Input: part model. Units: mm. Frame: model coordinates. A direction names the side the tool comes from. Give positions to 0.01 mm unless a question says otherwise; leave off trailing zeros. Loops run counter-clockwise (first coordinate to the right, second up) from the corner with the lowest first, then second, coordinate; pieces in that order, holes last. Notation, with made-up numbers: M -3,54.25 L 48,54.25 A19 ccw 48,78.25 Z; hole C 9.5,22 d10. An arc over 180 degrees is marked long. Answer as a JSON object with one key per item and string values. Group by question number.
1) Section query D-D on x = -26. Return loops of the section in (y, z), plus the area to 3 significant figures.
2) First-contact query: P1, Ø6, axis at x = -50, z = 0, coming from the -Y side; P2, Ø4, axis at x = -20, z = 0, coming from the +Y side; P3, Ø3, axis at y = -20, z = 0, coming from the +X side. Flat tips, straight axial feed; report the tip coordinate or a pass-through.
3) Ray query, L1, parallel to Y at x = -10.5, z = 0; L2, parallel to Z at x = -20, y = -8.5; L3, parallel to Y at x = -9, z = -1.75. Return the intervals inside material, ascending.
4) Section query C-C on x = -32.5. Return loops of the section in (y, z), plus the area to 4 significant figures.
5) Section query B-B on z = 4. Return loops of the section in (x, y), plus the area to 3 significant figures.
6) Access query for faces 4 (the cylindrical face through (-7.6, -42.56, 0.54)), 5 (the flat face through (-40, -50, 0)), 6 (the cylindrical face through (-17.5, -7.6, -0.1)). Directions: +Z, -Z, +X, -X, +Y, -Y. A direction counts if a zero-diameter tool reaches every point of the face in a straight line with its end or side. Return the directions, or none.
7) Section query A-A on y = -7. Return loops of the section in (x, z), plus the area to 3 significant figures.
8) Draft query along Z for faces 1 (the flat face through (0, -30, 0)), 2 (the cylindrical face through (-7.6, -22.48, 0.33)), 3 (the flat face through (-30, -30, -5)). Return one class per face: +Z half, -Z half, draft (parallel to the pull), parting line (faces both ways), or undercut.
from build123d import *

# Parameters (mm, degrees)
EXTRUDE_1_DEPTH        = 5
HOLE_WIZARD_M6_1_D     = 5
HOLE_WIZARD_M6_1_DEPTH = 15
HOLE_WIZARD_M6_1_TIP   = 1.502151548
HOLE_WIZARD_M6_2_D     = 5
HOLE_WIZARD_M6_2_DEPTH = 15
HOLE_WIZARD_M6_2_TIP   = 1.502151548


with BuildPart() as part:
    # 草图1 → 凸台-拉伸1 (new body, symmetric)
    with BuildSketch(Plane.XY):
        Polygon((0, 0), (-60, 0), (-60, -40), (-20, -60), (0, -60), align=None)
    extrude(amount=EXTRUDE_1_DEPTH, both=True)

    # M6 螺纹孔1
    with Locations(Plane(origin=(0, -20, 0), x_dir=(0, 0, 1), z_dir=(1, 0, 0))):
        with Locations((0, 0), (0, 25)):
            Hole(HOLE_WIZARD_M6_1_D / 2, depth=HOLE_WIZARD_M6_1_DEPTH)
            with Locations((0, 0, -(HOLE_WIZARD_M6_1_DEPTH + HOLE_WIZARD_M6_1_TIP / 2))):  # 118° drill point
                Cone(0, HOLE_WIZARD_M6_1_D / 2, HOLE_WIZARD_M6_1_TIP, mode=Mode.SUBTRACT)

    # M6 螺纹孔2
    with Locations(Plane(origin=(-20, 0, 0), x_dir=(1, 0, 0), z_dir=(0, 1, 0))):
        with Locations((0, 0), (-30, 0)):
            Hole(HOLE_WIZARD_M6_2_D / 2, depth=HOLE_WIZARD_M6_2_DEPTH)
            with Locations((0, 0, -(HOLE_WIZARD_M6_2_DEPTH + HOLE_WIZARD_M6_2_TIP / 2))):  # 118° drill point
                Cone(0, HOLE_WIZARD_M6_2_D / 2, HOLE_WIZARD_M6_2_TIP, mode=Mode.SUBTRACT)


solid = part.part
Output:
{
 "1": {"outline": "M -57,-5 L 0,-5 L 0,5 L -57,5 Z", "area": "570 mm^2"},
 "2": {"P1": "stops at y = -46.5", "P2": "stops at y = -15.3", "P3": "stops at x = -15.6"},
 "3": {"L1": "y = -60 to -47.5, -42.5 to -22.5, -17.5 to 0", "L2": "z = -5 to -2.5, 2.5 to 5", "L3": "y = -60 to -46.79, -43.21 to -21.79, -18.21 to 0"},
 "4": {"outline": "M -53.75,-5 L 0,-5 L 0,5 L -53.75,5 Z", "area": "537.5 mm^2"},
 "5": {"outline": "M -60,-40 L -20,-60 L 0,-60 L 0,0 L -60,0 Z", "area": "3,200 mm^2"},
 "6": {"face 4": "+X", "face 5": "+Z, -Z, -X, -Y", "face 6": "+Y"},
 "7": {"outline": "M -60,-5 L 0,-5 L 0,5 L -60,5 Z; hole C -50,0 d5; hole C -20,0 d5", "area": "561 mm^2"},
 "8": {"face 1": "draft", "face 2": "undercut", "face 3": "-Z half"}
}
